Here's how the part is built. I have some questions about the finished solid (model axes, mm). Face numbers are marked on the shaded views. Coordinates: 2 decimals unless noted, no trailing zeros. Write each loop counter-clockwise with the first axis right and the second up, starting at its lowest first coordinate (ties: lowest second). Pieces come first, ordered by that corner, then holes. Notation, with made-up numbers: (-16.5, 28.5) - (32.5, 28.5) arc R32 ccw to (32.5, 67.5) - close; hole circle Ø8 at (-12, -3.5). An arc over 180 degrees is marked (long way). Answer in a Markdown table with one row per item. Add a question column.
Item 1: We'd pull the mould along X, two halves only. Please class the marked faces 1, 2 and 3: +X half, -X half, draft (parallel to the pull), parting line (faces both ways), or undercut.
Item 2: If I drill on probe 1 along X at (y, z) = (2.5, 6); probe 2 along X at (y, z) = (-2.75, 7.75); probe 3 along X at (y, z) = (1.5, 8.75), over which ranges is the centre line in solid material (lowest first)? Write a range as from..to.
Item 3: I'm going to push a flat-ended pin straight in: pin 1 (1 mm diameter, centred on x = -1.5, y = 1, fed in from +Z). Where does the tip first touch, or does it pass through?
Item 4: Imagine slicing it at A-A (z = 7.75). Please give me the cut outline in (x, y), plus the area to 3 significant figures.
Item 5: Imagine slicing it at C-C (x = 1). Please give me the cut outline in (y, z), plus the area to 3 significant figures.
Item 6: Imagine slicing it at D-D (z = 9). Please give me the cut outline in (x, y).
Item 7: Imagine slicing it at B-B (y = 0.5). Please give me the cut outline in (x, z).
from build123d import *

# Parameters (mm, degrees)
F0_W     = 10
F0_H     = 14
F1_DEPTH = 10
F2_R     = 3
F3_DEPTH = 14.001


with BuildPart() as f1:
    # F0 (on Top) → F1 (new body)
    with BuildSketch(Plane.XY):
        Rectangle(F0_W, F0_H)
    extrude(amount=F1_DEPTH)

    # F2 (on face) → F3 (cut, through all)
    with BuildSketch(Plane.XZ.offset(7)):
        with Locations((0, 5)):
            Circle(F2_R)
        with BuildLine():
            ThreePointArc((-5, 5), (-3.535534, 8.535534), (0, 10))
            Line((0, 10), (-5, 10))
            Line((-5, 10), (-5, 5))
        make_face()
        with BuildLine():
            Line((5, 10), (0, 10))
            ThreePointArc((0, 10), (3.535534, 8.535534), (5, 5))
            Line((5, 5), (5, 10))
        make_face()
    extrude(amount=-F3_DEPTH, mode=Mode.SUBTRACT)


solid = f1.part
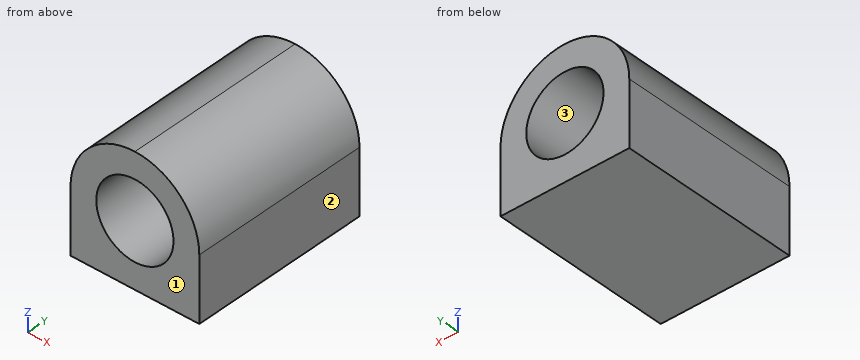
Here are the results:
| question | item | result |
|---|---|---|
| 1 | face 1 | draft |
| 1 | face 2 | +X half |
| 1 | face 3 | undercut |
| 2 | probe 1 | x = -4.9..-2.83, 2.83..4.9 |
| 2 | probe 2 | x = -4.18..-1.2, 1.2..4.18 |
| 2 | probe 3 | x = -3.31..3.31 |
| 3 | pin 1 | stops at z = 9.9 |
| 4 | outline | (-4.18, -7) - (-1.2, -7) - (-1.2, 7) - (-4.18, 7) - close; (1.2, -7) - (4.18, -7) - (4.18, 7) - (1.2, 7) - close |
| 4 | area | 83.4 mm2 |
| 5 | outline | (-7, 0) - (7, 0) - (7, 2.17) - (-7, 2.17) - close; (-7, 7.83) - (7, 7.83) - (7, 9.9) - (-7, 9.9) - close |
| 5 | area | 59.4 mm2 |
| 6 | outline | (-3, -7) - (3, -7) - (3, 7) - (-3, 7) - close |
| 7 | outline | (-5, 0) - (5, 0) - (5, 5) arc R5 ccw to (-5, 5) - close; hole circle Ø6 at (0, 5) |
